from build123d import *

# Parameters (mm, degrees)
F0_R     = 63.5
F1_DEPTH = 254
F4_R     = 5.08
F5_W     = 50.8
F5_H     = 50.8
F6_DEPTH = 76.2


# Not quite as in the source:
# - the program builds the solid bodies; features that only make, move or delete a surface that nothing else refers to are left out


with BuildPart() as f1:
    # F0 (on Front) → F1 (new body)
    with BuildSketch(Plane.XZ):
        Circle(F0_R)
    extrude(amount=F1_DEPTH)

    # F4
    f4_edges = [f1.edges().sort_by_distance(p)[0] for p in [
        (-63.5, -254, 0),
        (-63.5, 0, 0),
    ]]
    fillet(f4_edges, radius=F4_R)

    # F5 (on Top) → F6 (join)
    with BuildSketch(Plane.XY):
        with Locations((0, -47.7578863502)):
            Rectangle(F5_W, F5_H)
    extrude(amount=-F6_DEPTH)


solid = f1.part
Input: part model. Units: mm. Frame: model coordinates. A direction names the side the tool comes from. Coordinates: 2 decimals unless noted, no trailing zeros. Loops run counter-clockwise (first coordinate to the right, second up) from the corner with the lowest first, then second, coordinate; pieces in that order, holes last.
(1) Section A-A on x = 0. Return the cut outline in (y, z).
(2) Section C-C on y = -61.5. Return the cut outline in (x, z).
(3) Section B-B on y = -135. Return the cut outline in (x, z).
(4) First-contact query: pin 1 Ø20 at (y, z) = (-57, -65.5) entering from +X; pin 2 Ø1.5 at (x, y) = (-32.5, -198) entering from +Z; pin 3 Ø1 at (y, z) = (-127, 7) entering from +X. Flat tips, straight axial feed; report the tip coordinate or a pass-through.
(5) Material intervals for probe 1 along Y at (x, z) = (53, 30); probe 2 along X at (y, z) = (-43, 23); probe 3 along X at (y, z) = (-149.5, 50), sorted ascending.
(6) Set-up query: faces 1 (the face through (25.4, -48, -67)), 2 (the face through (0, -47, -76.2)), 3 (the face through (-25.4, -48, -67)). Return all of +Z, -Z, +X, -X, +Y, -Y with unobstructed straight access to the full face (end or side cutting, diameter ignored); none if empty.
Data:
1. outline: (-254, -58.42) arc R5.08 ccw to (-248.92, -63.5) - (-73.16, -63.5) - (-73.16, -76.2) - (-22.36, -76.2) - (-22.36, -63.5) - (-5.08, -63.5) arc R5.08 ccw to (0, -58.42) - (0, 58.42) arc R5.08 ccw to (-5.08, 63.5) - (-248.92, 63.5) arc R5.08 ccw to (-254, 58.42) - close
2. outline: (-25.4, -76.2) - (25.4, -76.2) - (25.4, -58.2) arc R63.5 ccw (long way) to (-25.4, -58.2) - close
3. outline: circle Ø127 at (0, 0)
4. pin 1: stops at x = 30.85
4. pin 2: stops at z = 54.99
4. pin 3: stops at x = 63.17
5. probe 1: y = -253.35 to -0.65
5. probe 2: x = -59.19 to 59.19
5. probe 3: x = -39.14 to 39.14
6. face 1: -Z, +X, +Y, -Y
6. face 2: -Z, +X, -X, +Y, -Y
6. face 3: -Z, -X, +Y, -Y
